Check sheet for the drawn part. Datum: minimum x, y, z corner. Units: mm. A direction names the side the tool comes from. Coordinates: 2 decimals unless noted, no trailing zeros. Write each loop counter-clockwise with the first axis right and the second up, starting at its lowest first coordinate (ties: lowest second). Pieces come first, ordered by that corner, then holes. Notation, with made-up numbers: (48.5, 21.25) - (106.5, 21.25) arc R9 ccw to (106.5, 29.25) - close; hole circle Ø2 at (60, 42). An arc over 180 degrees is marked (long way). Write each question's results on one line, items separated by ' | '.
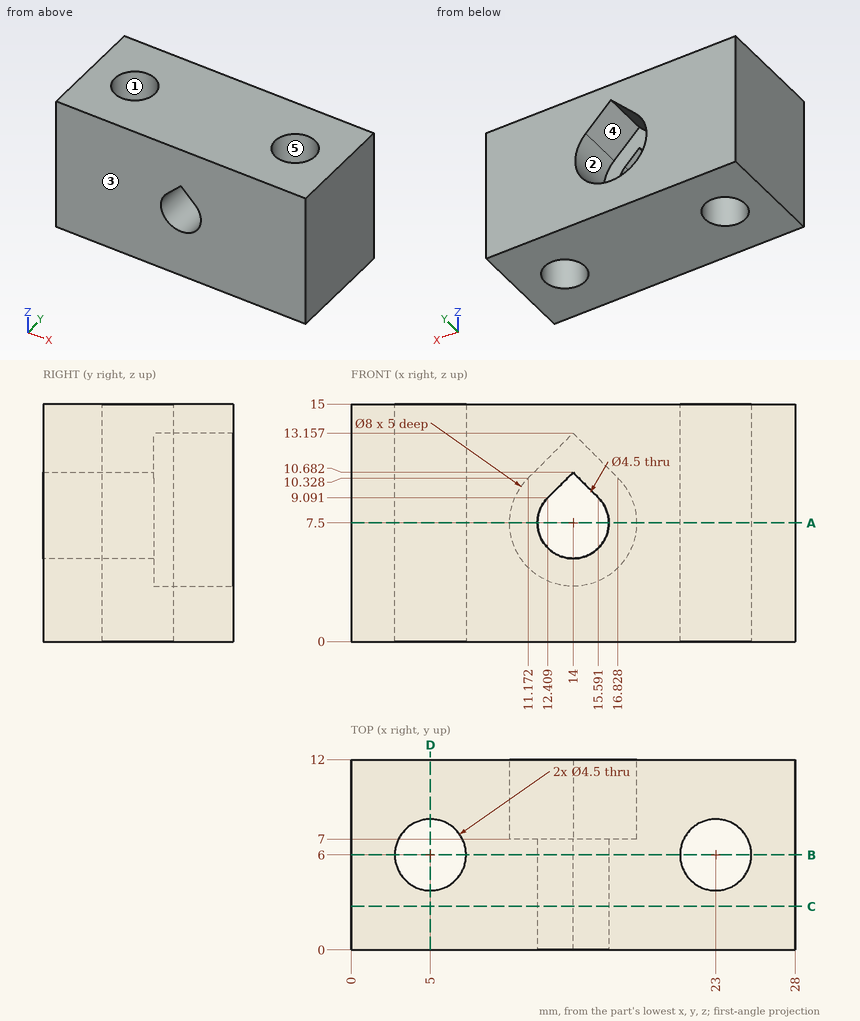
1. Sectioned sample at D-D (x = 5). Record the cut outline in (y, z).
Values follow:
outline: (0, 0) - (3.75, 0) - (3.75, 15) - (0, 15) - close; (8.25, 0) - (12, 0) - (12, 15) - (8.25, 15) - close
2. Access from +Z, -Z, +X, -X, +Y, -Y to the whole of each face (thin tool, end or side, straight path). Record for the marked faces 4 and 5.
Values follow:
face 4: +Y | face 5: +Z, -Z
3. Material ranges on L1, parallel to X at y = 2.25, z = 7.5; L2, parallel to Y at x = 23, z = 9.25; L3, parallel to X at y = 5, z = 9.75 (1 decimal), recorded low to high. Write a range as [from, to].
Values follow:
L1: x = [0, 11.75], [16.25, 28] | L2: y = [0, 3.75], [8.25, 12] | L3: x = [0, 3], [7, 13.1], [14.9, 21], [25, 28]
4. Sectioned sample at B-B (y = 6). Record the cut outline in (x, z), then the cut area to 3 significant figures.
Values follow:
outline: (0, 0) - (2.75, 0) - (2.75, 15) - (0, 15) - close; (7.25, 0) - (20.75, 0) - (20.75, 15) - (7.25, 15) - close; (25.25, 0) - (28, 0) - (28, 15) - (25.25, 15) - close; hole (12.41, 9.09) arc R2.25 ccw (long way) to (15.59, 9.09) - (14, 10.68) - close | area: 268 mm^2
5. Sectioned sample at C-C (y = 2.75). Record the cut outline in (x, z).
Values follow:
outline: (0, 0) - (28, 0) - (28, 15) - (0, 15) - close; hole (12.41, 9.09) arc R2.25 ccw (long way) to (15.59, 9.09) - (14, 10.68) - close
6. Go/stop test with a flat-tipped pin: pin 1 (7 mm diameter, centred on x = 14, z = 7.5, fed in from +Y). Record where the tip stops, or that it passes through.
Values follow:
pin 1: stops at y = 7
7. Sectioned sample at A-A (z = 7.5). Record the cut outline in (x, y), then the cut area to 3 significant figures.
Values follow:
outline: (0, 0) - (11.75, 0) - (11.75, 7) - (10, 7) - (10, 12) - (0, 12) - close; (16.25, 0) - (28, 0) - (28, 12) - (18, 12) - (18, 7) - (16.25, 7) - close; hole circle Ø4.5 at (5, 6); hole circle Ø4.5 at (23, 6) | area: 233 mm^2
8. Draft check along Y on the marked faces 1, 2 and 3. Enter one of: pulls with the +Y half, pulls with the -Y half, needs draft (parallel to the pull), parting line crosses it, or undercut.
Values follow:
face 1: undercut | face 2: needs draft | face 3: pulls with the -Y half
